Geometry check sheet. Reference: the model listing, model coordinates, mm. A direction names the side the tool comes from. Coordinates: 2 decimals unless noted, no trailing zeros. Order: outer loops, then holes, each group sorted by start corner. A loop starts at its lowest first (then second) coordinate and runs counter-clockwise, first axis right, second up. Notation, with made-up numbers: (34, 53) - (59, 53) arc R15 cw to (59, 74) - close; hole circle Ø7 at (76, 53.25). An arc over 180 degrees is marked (long way). Return JSON: item names as keys, results as strings. Group by question number.
Item 1: Tool access check on faces 4 (the flat face through (5.09, 2.94, 5.51)), 5 (the cylindrical face through (-6.246, 0.229, 11.381)), 6 (the flat face through (-4, 4, 0)). Record the directions out of +Z, -Z, +X, -X, +Y, -Y that give a thin tool (end or side, any length) a straight path to the whole face; none if there is none.
Item 2: Draft check along Y on faces 1 (the flat face through (15, 12, 1)), 2 (the cylindrical face through (-4.13, 0.15, 1.48)), 3 (the flat face through (0, -15, 1)). Enter one of: pulls with the +Y half, pulls with the -Y half, needs draft (parallel to the pull), parting line crosses it, or undercut.
Item 3: Scan lines: probe 1 along Y at (x, z) = (0, 0.9); probe 2 along Y at (x, z) = (0, 10.5); probe 3 along Z at (x, y) = (-9, -0.25). Record each from-to range of solid material in increasing order.
Item 4: Section check B-B on y = 0. Enter the section's corners in (x, z).
Item 5: Section check D-D on z = 17.75. Enter the section's corners in (x, y) (3 decimals), then the cut area to 3 significant figures.
Item 6: Gauge pin test, flat ends, axial feed: pin 1 (15 mm diameter, centred on x = 0, y = -4, fed in from +Z); pin 2 (1.5 mm diameter, centred on x = 5, z = 8.5, fed in from +Y); pin 3 (6 mm diameter, centred on y = -5.5, z = 16.5, fed in from -X); pin 4 (1.5 mm diameter, centred on x = -8, y = -7.5, fed in from +Z). Record the tip position at first contact, or that the pin passes through.
Item 7: Section check A-A on x = 11.5. Enter the section's corners in (y, z), then the cut area to 3 significant figures.
Item 8: Section check C-C on x = 0. Enter the section's corners in (y, z), then the cut area to 3 significant figures.
from build123d import *

# Parameters (mm, degrees)
F0_R     = 6.25
F0_R_2   = 4.25
F1_DEPTH = 20
F2_W     = 30
F2_H     = 30
F3_DEPTH = 3
F4_R     = 4.134278
F5_DEPTH = 20.001
F7_DEPTH = 25


with BuildPart() as f1:
    # F0 (on Top) → F1 (new body)
    with BuildSketch(Plane.XY):
        Circle(F0_R)
        Circle(F0_R_2, mode=Mode.SUBTRACT)
    extrude(amount=F1_DEPTH)

    # F2 (on Top) → F3 (join)
    with BuildSketch(Plane.XY):
        Rectangle(F2_W, F2_H)
    extrude(amount=F3_DEPTH)

    # F4 (on Top) → F5 (cut, through all)
    with BuildSketch(Plane.XY):
        Circle(F4_R)
    extrude(amount=F5_DEPTH, mode=Mode.SUBTRACT)

    # F6 (on Top) → F7 (cut)
    with BuildSketch(Plane.XY):
        Polygon((63.665008, -36.75701), (63.665008, 36.75701), (0, 0), align=None)
    extrude(amount=F7_DEPTH, mode=Mode.SUBTRACT)


solid = f1.part
Computed:
{
 "1": {"face 4": "+Z, -Z, +X", "face 5": "+Z", "face 6": "-Z, +X, -X, +Y, -Y"},
 "2": {"face 1": "needs draft", "face 2": "undercut", "face 3": "pulls with the -Y half"},
 "3": {"probe 1": "y = -15 to -4.13, 4.13 to 15", "probe 2": "y = -6.25 to -4.25, 4.25 to 6.25", "probe 3": "z = 0 to 3"},
 "4": {"outline": "(-15, 0) - (-4.13, 0) - (-4.13, 3) - (-4.25, 3) - (-4.25, 20) - (-6.25, 20) - (-6.25, 3) - (-15, 3) - close"},
 "5": {"outline": "(3.681, -2.125) arc R4.25 cw (long way) to (3.681, 2.125) - (5.413, 3.125) arc R6.25 ccw (long way) to (5.413, -3.125) - close", "area": "55.0 mm²"},
 "6": {"pin 1": "stops at z = 20", "pin 2": "stops at y = 4.58", "pin 3": "stops at x = -5.73", "pin 4": "stops at z = 3"},
 "7": {"outline": "(-15, 0) - (-6.64, 0) - (-6.64, 3) - (-15, 3) - close; (6.64, 0) - (15, 0) - (15, 3) - (6.64, 3) - close", "area": "50.2 mm²"},
 "8": {"outline": "(-15, 0) - (-4.13, 0) - (-4.13, 3) - (-4.25, 3) - (-4.25, 20) - (-6.25, 20) - (-6.25, 3) - (-15, 3) - close; (4.13, 0) - (15, 0) - (15, 3) - (6.25, 3) - (6.25, 20) - (4.25, 20) - (4.25, 3) - (4.13, 3) - close", "area": "133 mm²"}
}
